For this review, take the finished solid that the model builds, in its own axes (mm). Face numbers are marked on the shaded views. Coordinates: 2 decimals unless noted, no trailing zeros. Order: outer loops, then holes, each group sorted by start corner. A loop starts at its lowest first (then second) coordinate and runs counter-clockwise, first axis right, second up.
from build123d import *

# Parameters (mm, degrees)
F0_R     = 12.5
F0_R_2   = 7.5
F1_DEPTH = 100
F2_R     = 12.5
F3_DEPTH = 25
F4_R     = 5
F5_R     = 9
F5_R_2   = 7.5
F6_DEPTH = 25


with BuildPart() as f1:
    # F0 (on Top) → F1 (new body)
    with BuildSketch(Plane.XY):
        Circle(F0_R)
        Circle(F0_R_2, mode=Mode.SUBTRACT)
    extrude(amount=F1_DEPTH)

    # F2 (on face) → F3 (join)
    with BuildSketch(Plane(origin=(0, 0, 0), x_dir=(1, 0, 0), z_dir=(0, 0, -1))):
        Circle(F2_R)
    extrude(amount=F3_DEPTH)

    # F4
    f4_edges = [f1.edges().sort_by_distance(p)[0] for p in [
        (-12.5, 0, -25),
        (-7.5, 0, 0),
    ]]
    fillet(f4_edges, radius=F4_R)

    # F5 (on face) → F6 (cut)
    with BuildSketch(Plane.XY.offset(100)):
        Circle(F5_R)
        Circle(F5_R_2, mode=Mode.SUBTRACT)
    extrude(amount=-F6_DEPTH, mode=Mode.SUBTRACT)


solid = f1.part
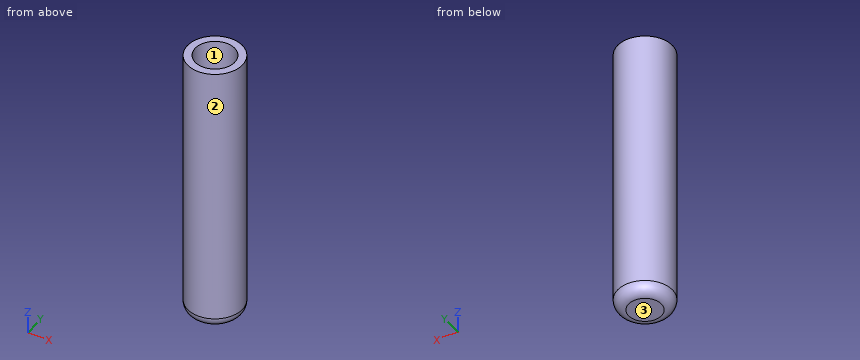
1. Take a section at A-A, the plane z = 34. Give the boundary of the cut face in (x, y).
Answer below:
outline: circle Ø25 at (0, 0); hole circle Ø15 at (0, 0)
2. Take a section at B-B, the plane z = -2.5. Give the boundary of the cut face in (x, y), plus the area to 3 significant figures.
Answer below:
outline: circle Ø25 at (0, 0)
area: 491 mm2
3. To check wall thickness, follow L1, parallel to Y at x = 0, z = 82.25; L2, parallel to Y at x = 0, z = 37.5; L3, parallel to X at y = 2.75, z = 14.5. State the ranges of each line that lie inside material, in increasing order.
Answer below:
L1: y = -12.5 to -9, 9 to 12.5
L2: y = -12.5 to -7.5, 7.5 to 12.5
L3: x = -12.19 to -6.98, 6.98 to 12.19
4. Clearance check with flat-ended pins moving along their axes: pin 1 Ø1.5 at (x, z) = (4, 83.5) entering from -Y; pin 2 Ø12 at (x, z) = (-7, 49.5) entering from +Y; pin 3 Ø5.5 at (x, y) = (1, -1) entering from +Z. State where each tip first meets the part, or that it passes through.
Answer below:
pin 1: stops at y = -12.07
pin 2: stops at y = 12.46
pin 3: stops at z = 0.29
5. The part is to be moulded in two halves that separate along Y. For the marked faces 1, 2 and 3, say which applies: +Y half, -Y half, draft (parallel to the pull), parting line (faces both ways), or undercut.
Answer below:
face 1: undercut
face 2: parting line
face 3: draft
